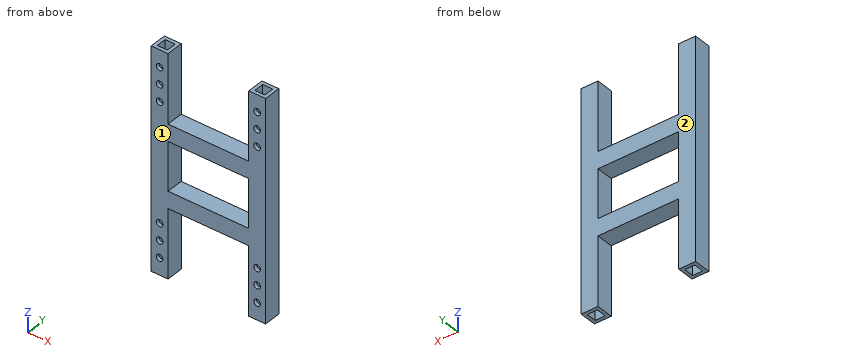
from build123d import *

# Parameters (mm, degrees)
SKETCH1_W               = 50
SKETCH1_H               = 50
SKETCH1_W_2             = 30
SKETCH1_H_2             = 30
BOSS_EXTRUDE1_DEPTH     = 650
BOSS_EXTRUDE1_2_DEPTH   = 650
SKETCH2_R               = 10
CUT_EXTRUDE1_DEPTH      = 18
CUT_EXTRUDE1_DEPTH_BACK = 13
SKETCH3_W               = 50
SKETCH3_H               = 50
SKETCH3_W_2             = 30
SKETCH3_H_2             = 30
BOSS_EXTRUDE3_DEPTH     = 240


with BuildPart() as part:
    # Sketch1 → Boss-Extrude1 (new body)
    with BuildSketch(Plane.XY):
        Rectangle(SKETCH1_W, SKETCH1_H)
        Rectangle(SKETCH1_W_2, SKETCH1_H_2, mode=Mode.SUBTRACT)
    extrude(amount=BOSS_EXTRUDE1_DEPTH)


with BuildPart() as body_2:
    # Sketch1 → Boss-Extrude1 2 (new body)
    with BuildSketch(Plane.XY):
        with Locations((290, 0)):
            Rectangle(SKETCH1_W, SKETCH1_H)
        with Locations((290, 0)):
            Rectangle(SKETCH1_W_2, SKETCH1_H_2, mode=Mode.SUBTRACT)
    extrude(amount=BOSS_EXTRUDE1_2_DEPTH)


with BuildPart() as cut_extrude1_tool:
    # Sketch2 → Cut-Extrude1 (new body, two sides)
    with BuildSketch(Plane.XZ.offset(25)) as cut_extrude1_sk:
        with Locations((290, 600)):
            Circle(SKETCH2_R)
        with Locations((290, 550)):
            Circle(SKETCH2_R)
        with Locations((290, 500)):
            Circle(SKETCH2_R)
        with Locations((290, 150)):
            Circle(SKETCH2_R)
        with Locations((290, 100)):
            Circle(SKETCH2_R)
        with Locations((290, 50)):
            Circle(SKETCH2_R)
        with Locations((0, 500)):
            Circle(SKETCH2_R)
        with Locations((0, 550)):
            Circle(SKETCH2_R)
        with Locations((0, 600)):
            Circle(SKETCH2_R)
        with Locations((0, 50)):
            Circle(SKETCH2_R)
        with Locations((0, 100)):
            Circle(SKETCH2_R)
        with Locations((0, 150)):
            Circle(SKETCH2_R)
    extrude(amount=CUT_EXTRUDE1_DEPTH)
    extrude(cut_extrude1_sk.sketch, amount=-CUT_EXTRUDE1_DEPTH_BACK)


with BuildPart() as part_1:
    add(part.part)

    # Cut-Extrude1: cut by cut_extrude1_tool
    add(cut_extrude1_tool.part, mode=Mode.SUBTRACT)



with BuildPart() as body_2_1:
    add(body_2.part)

    # Cut-Extrude1: cut by cut_extrude1_tool
    add(cut_extrude1_tool.part, mode=Mode.SUBTRACT)


with BuildPart() as part_2:
    add(part_1.part)

    add(body_2_1.part)  # Boss-Extrude3 merges body 2
    # Sketch3 → Boss-Extrude3 (add)
    with BuildSketch(Plane.ZY.offset(-265)):
        with Locations((421.770995298, 0)):
            Rectangle(SKETCH3_W, SKETCH3_H)
        with Locations((421.770995298, 0)):
            Rectangle(SKETCH3_W_2, SKETCH3_H_2, mode=Mode.SUBTRACT)
        with Locations((228.229004702, 0)):
            Rectangle(SKETCH3_W, SKETCH3_H)
        with Locations((228.229004702, 0)):
            Rectangle(SKETCH3_W_2, SKETCH3_H_2, mode=Mode.SUBTRACT)
    extrude(amount=BOSS_EXTRUDE3_DEPTH)


solid = part_2.part
Could you check a few things on this model? Use its own coordinates, in mm. Face numbers are marked on the shaded views. Coordinates: 2 decimals unless noted, no trailing zeros. Loops run counter-clockwise (first coordinate to the right, second up) from the corner with the lowest first, then second, coordinate; pieces in that order, holes last.
1. Imagine slicing it at A-A (z = 342.5). Please give me the cut outline in (x, y), and give its area (3 significant figures).
2. Imagine slicing it at C-C (y = 3). Give the number of separate pieces and of enclosed holes in the cut face, and give its area (3 significant figures).
3. I need wall thicknesses on L1, parallel to X at y = 5.5, z = 603.5; L2, parallel to Z at x = 28.5, y = -0.5; L3, parallel to Z at x = 73, y = 16. Which ranges of each line are inside material? Lowest first, please.
4. Imagine slicing it at D-D (z = 500). Please give me the cut outline in (x, y), and give its area (3 significant figures).
5. Imagine slicing it at B-B (x = 222.5). Please give me the cut outline in (y, z), and give its area (3 significant figures).
6. For P1, Ø25, axis at x = 188.5, y = -9, coming from the +Z side; P2, Ø18, axis at x = 290, z = 550, coming from the -Y side; P3, Ø24, axis at x = 146.5, y = -2, coming from the -Z side, each with a flat end and sliding along its axis, tell me the tip position at first contact or that it passes through.
7. We'd pull the mould along Y, two halves only. Please class the marked faces 1 and 2: released by +Y, released by -Y, zero draft, split by the parting line, or undercut.
Computed values:
1. outline: (-25, -25) - (25, -25) - (25, 25) - (-25, 25) - close; (265, -25) - (315, -25) - (315, 25) - (265, 25) - close; hole (-15, -15) - (15, -15) - (15, 15) - (-15, 15) - close; hole (275, -15) - (305, -15) - (305, 15) - (275, 15) - close
1. area: 3,200 mm2
2. separate pieces: 3
2. enclosed holes: 3
2. area: 35,600 mm2
3. L1: x = -25 to -15, 15 to 25, 265 to 275, 305 to 315
3. L2: z = 203.23 to 213.23, 243.23 to 253.23, 396.77 to 406.77, 436.77 to 446.77
3. L3: z = 203.23 to 253.23, 396.77 to 446.77
4. outline: (-25, -25) - (-10, -25) - (-10, -15) - (-15, -15) - (-15, 15) - (15, 15) - (15, -15) - (10, -15) - (10, -25) - (25, -25) - (25, 25) - (-25, 25) - close; (265, -25) - (280, -25) - (280, -15) - (275, -15) - (275, 15) - (305, 15) - (305, -15) - (300, -15) - (300, -25) - (315, -25) - (315, 25) - (265, 25) - close
4. area: 2,800 mm2
5. outline: (-25, 203.23) - (25, 203.23) - (25, 253.23) - (-25, 253.23) - close; (-25, 396.77) - (25, 396.77) - (25, 446.77) - (-25, 446.77) - close; hole (-15, 213.23) - (15, 213.23) - (15, 243.23) - (-15, 243.23) - close; hole (-15, 406.77) - (15, 406.77) - (15, 436.77) - (-15, 436.77) - close
5. area: 3,200 mm2
6. P1: stops at z = 446.77
6. P2: stops at y = 15
6. P3: stops at z = 203.23
7. face 1: released by -Y
7. face 2: released by +Y
